Geometry check sheet. Reference: the model listing, model coordinates, mm. Give positions to 0.01 mm unless a question says otherwise; leave off trailing zeros. Loops run counter-clockwise (first coordinate to the right, second up) from the corner with the lowest first, then second, coordinate; pieces in that order, holes last. Notation, with made-up numbers: (32, 11) -> (59, 11) arc R18 ccw to (59, 19) -> close; hole circle Ø2 at (26, 45). An arc over 180 degrees is marked (long way). Write item = value, one per line.
Autodesk Inventor part; units mm, degrees
ref_plane "YZ Plane" through (0, 0, 0) normal (1, 0, 0) x (0, 1, 0)
ref_plane "XZ Plane" through (0, 0, 0) normal (0, 1, 0) x (-1, 0, 0)
ref_plane "XY Plane" through (0, 0, 0) normal (0, 0, 1) x (1, 0, 0)
sketch "Sketch1" plane through (0, 0, 0) normal (0, 0, 1) x (1, 0, 0)
  line L0 (0, 0) -> (0, 15.875)
  line L1 (0, 15.875) -> (0.7937, 15.875)
  line L2 (0.7937, 15.875) -> (0.7938, 0.7937)
  line L3 (0.7938, 0.7937) -> (15.875, 0.7937)
  line L4 (15.875, 0.7937) -> (15.875, 0)
  line L5 (15.875, 0) -> (0, 0)
  dimension "d0" = 15.875
  dimension "d1" = 0.7937
extrude "Extrusion1" add sketch "Sketch1" along normal blind 107.95
sketch "Sketch2" plane through (0, 0, 0) normal (0, -1, 0) x (1, 0, 0)
  line L0 (15.875, 0) -> (0, 0)
  line L1 (0, 107.95) -> (15.875, 107.95)
  line L2 (7.9375, 107.95) -> (7.9375, 0) construction
  circle A0 centre (7.9375, 90.4875) radius 1.905
  circle A1 centre (7.9375, 9.525) radius 1.905
  line L3 (257.175, 98.425) -> (-9.525, 98.425) construction
  line L4 (-15.875, 82.55) -> (187.325, 82.55) construction
  dimension "d4" = 3.81
  dimension "d6" = 17.4625
  dimension "d7" = 9.525
  dimension "d16" = 15.875
  dimension "d17" = 9.525
extrude "Extrusion2" cut sketch "Sketch2" against normal through all
sketch "Sketch3" plane through (0, 0, 0) normal (-1, 0, 0) x (0, 0, 1)
  line L0 (0, 0) -> (0, 15.875)
  line L1 (107.95, 15.875) -> (107.95, 0)
  line L2 (0, 7.9375) -> (107.95, 7.9375) construction
  circle A0 centre (9.525, 7.9375) radius 1.905
  circle A1 centre (98.425, 7.9375) radius 1.905
  dimension "d11" = 3.81
  dimension "d12" = 9.525
  dimension "d13" = 9.525
extrude "Extrusion3" cut sketch "Sketch3" against normal through all
equation "\"d6\" = d17 + 0.5 * d16"
properties part number "Hopper Bracing P2" material "Aluminum 6061"
Item 1: Section check C-C, the plane y = 14.5. Record the cut outline in (x, z), plus the area to 3 significant figures.
Answer:
outline = (0, 0) -> (0.79, 0) -> (0.79, 107.95) -> (0, 107.95) -> close
area = 85.7 mm^2
Item 2: Thickness scan on L1, parallel to X at y = 1.75, z = 29.5. Record the ranges inside material, lowest first. Write a range as [from, to].
Answer:
L1 = [0, 0.79]
Item 3: Section check A-A, the plane x = 8.5. Record the cut outline in (y, z), plus the area to 3 significant figures.
Answer:
outline = (0, 0) -> (0.79, 0) -> (0.79, 7.7) -> (0, 7.7) -> close; (0, 11.35) -> (0.79, 11.35) -> (0.79, 88.67) -> (0, 88.67) -> close; (0, 92.31) -> (0.79, 92.31) -> (0.79, 107.95) -> (0, 107.95) -> close
area = 79.9 mm^2
Item 4: Draft check along X on faces 1 (the flat face through (8, 0.794, 53)), 2 (the flat face through (0, 8, 53)), 3 (the cylindrical face through (7.69, 0.391, 92.376)), 4 (the cylindrical face through (8.96, 0.39, 11.13)). Enter one of: +X half, -X half, draft (parallel to the pull), parting line (faces both ways), or undercut.
Answer:
face_1 = draft
face_2 = -X half
face_3 = undercut
face_4 = undercut
Item 5: Section check B-B, the plane z = 15. Record the cut outline in (x, y) (3 decimals).
Answer:
outline = (0, 0) -> (15.875, 0) -> (15.875, 0.794) -> (0.794, 0.794) -> (0.794, 15.875) -> (0, 15.875) -> close
Item 6: Gauge pin test, flat ends, axial feed: pin 1 (4.5 mm diameter, centred on x = 9.5, z = 50, fed in from +Y); pin 2 (4.5 mm diameter, centred on y = 7.5, z = 70.5, fed in from +X); pin 3 (2.5 mm diameter, centred on y = 7.94, z = 9.52, fed in from +X). Record the tip position at first contact, or that the pin passes through.
Answer:
pin_1 = 0.79
pin_2 = 0.79
pin_3 = through
